CAD build for the part. Positions are in the model's coordinates, mm. Coordinates: 2 decimals unless noted, no trailing zeros. Loops run counter-clockwise (first coordinate to the right, second up) from the corner with the lowest first, then second, coordinate; pieces in that order, holes last. Notation, with made-up numbers: (67.25, 43.25) -> (110.25, 43.25) arc R12 ccw to (110.25, 62.25) -> close; hole circle Ø10 at (-35, -4.5). An arc over 180 degrees is marked (long way). Write each question's results on one line, items separated by ' | '.
```python
from build123d import *

# Parameters (mm, degrees)
F0_W     = 59
F0_H     = 59
F1_DEPTH = 29.5
F2_R     = 16.5
F3_DEPTH = 29.501
F4_W     = 59
F4_H     = 29.5
F5_DEPTH = 29.501


with BuildPart() as f1:
    # F0 (on Front) → F1 (new body)
    with BuildSketch(Plane.XZ):
        Rectangle(F0_W, F0_H)
    extrude(amount=F1_DEPTH)

    # F2 (on face) → F3 (cut, through all)
    with BuildSketch(Plane.XZ.offset(29.5)):
        Circle(F2_R)
    extrude(amount=-F3_DEPTH, mode=Mode.SUBTRACT)

    # F4 (on face) → F5 (cut, through all)
    with BuildSketch(Plane(origin=(0, 0, 0), x_dir=(-1, 0, 0), z_dir=(0, 1, 0))):
        with Locations((0, 14.75)):
            Rectangle(F4_W, F4_H)
    extrude(amount=-F5_DEPTH, mode=Mode.SUBTRACT)


solid = f1.part
```
Q1. Cut at B-B on y = -10. Write the cut outline in (x, z).
Results are:
outline: (-29.5, -29.5) -> (29.5, -29.5) -> (29.5, 0) -> (16.5, 0) arc R16.5 cw to (-16.5, 0) -> (-29.5, 0) -> close
Q2. Cut at D-D on z = -9.75. Write the cut outline in (x, y), and give its area (3 significant figures).
Results are:
outline: (-29.5, -29.5) -> (-13.31, -29.5) -> (-13.31, 0) -> (-29.5, 0) -> close; (13.31, -29.5) -> (29.5, -29.5) -> (29.5, 0) -> (13.31, 0) -> close | area: 955 mm^2
Q3. Cut at C-C on x = 0. Write the cut outline in (y, z).
Results are:
outline: (-29.5, -29.5) -> (0, -29.5) -> (0, -16.5) -> (-29.5, -16.5) -> close
Q4. Wall check: L1, parallel to X at y = -2.25, z = -13.5; L2, parallel to X at y = -27.5, z = -6.5; L3, parallel to Z at x = 14, y = -3.75. Give the ranges that are in metal, low to high. Write a range as from..to.
Results are:
L1: -29.5..-9.49, 9.49..29.5 | L2: -29.5..-15.17, 15.17..29.5 | L3: -29.5..-8.73
Q5. Cut at A-A on z = -4.25. Write the cut outline in (x, y).
Results are:
outline: (-29.5, -29.5) -> (-15.94, -29.5) -> (-15.94, 0) -> (-29.5, 0) -> close; (15.94, -29.5) -> (29.5, -29.5) -> (29.5, 0) -> (15.94, 0) -> close
